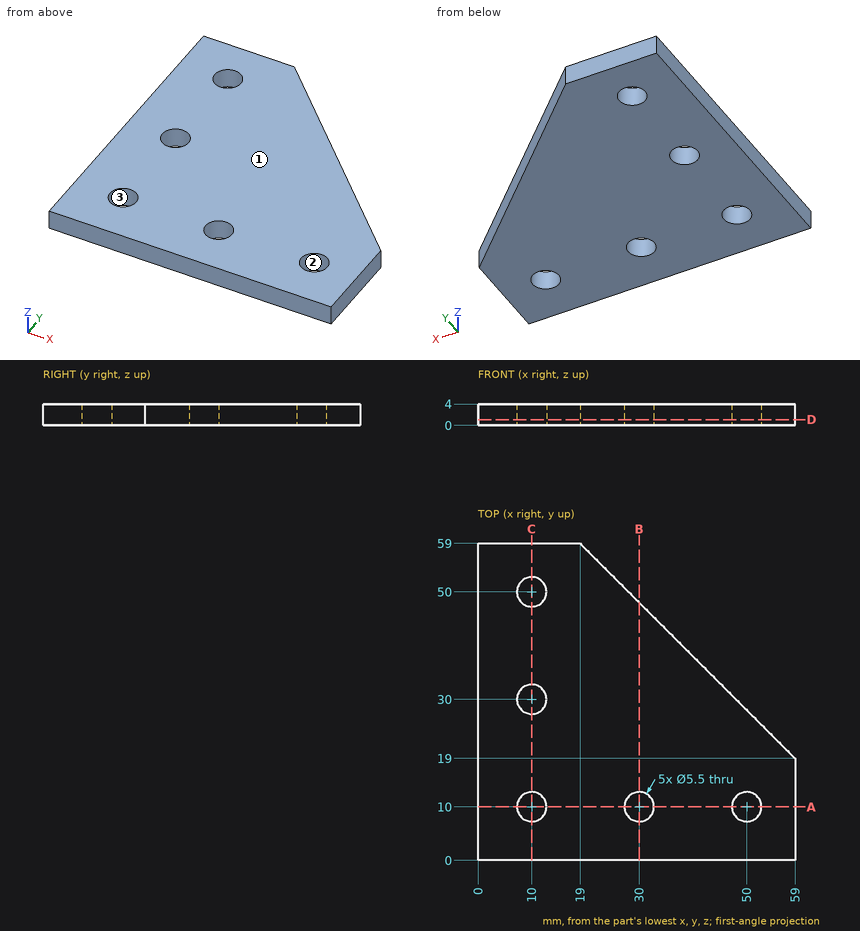
Here's the drawing with two shaded views (mm, measured from the low corner). I have some questions. Give positions to 0.01 mm unless a question says otherwise; leave off trailing zeros. Loops run counter-clockwise (first coordinate to the right, second up) from the corner with the lowest first, then second, coordinate; pieces in that order, holes last. Notation, with made-up numbers: (59, 37.25) - (96, 37.25) arc R24 cw to (96, 72.25) - close; hole circle Ø2 at (55.25, 82). An arc over 180 degrees is marked (long way). One line per item, written item: value.
(1) If we section it at B-B, the plane x = 30: List the corners of the cut face in (y, z) for me, plus the area to 3 significant figures.
Verdict:
outline: (0, 0) - (7.25, 0) - (7.25, 4) - (0, 4) - close; (12.75, 0) - (48, 0) - (48, 4) - (12.75, 4) - close
area: 170 mm^2
(2) If we mould it in two halves opening along X, with no side actions, what happens to the marked faces 1, 2 and 3? For each: released by +X, released by -X, zero draft, split by the parting line, or undercut.
Verdict:
face 1: zero draft
face 2: undercut
face 3: undercut
(3) I'm going to push flat-ended pins straight in: pin 1 (2 mm diameter, centred on x = 46, z = 2.5, fed in from -Y); pin 2 (4.5 mm diameter, centred on x = 30, y = 10, fed in from -Z). Where does each tip first touch, or does it pass through?
Verdict:
pin 1: y = 0
pin 2: through
(4) If we section it at A-A, the plane y = 10: List the corners of the cut face in (x, z) for me, plus the area to 3 significant figures.
Verdict:
outline: (0, 0) - (7.25, 0) - (7.25, 4) - (0, 4) - close; (12.75, 0) - (27.25, 0) - (27.25, 4) - (12.75, 4) - close; (32.75, 0) - (47.25, 0) - (47.25, 4) - (32.75, 4) - close; (52.75, 0) - (59, 0) - (59, 4) - (52.75, 4) - close
area: 170 mm^2
(5) If we section it at D-D, the plane z = 1.1: List the corners of the cut face in (x, y) for me.
Verdict:
outline: (0, 0) - (59, 0) - (59, 19) - (19, 59) - (0, 59) - close; hole circle Ø5.5 at (10, 10); hole circle Ø5.5 at (10, 30); hole circle Ø5.5 at (10, 50); hole circle Ø5.5 at (30, 10); hole circle Ø5.5 at (50, 10)
(6) I need wall thicknesses on line 1 along Y through (x, z) = (10, 1.5); line 2 along Y through (x, z) = (9, 3.4); line 3 along Y through (x, z) = (50, 2.55). Which ranges of each line are inside material? Lowest first, please.
Verdict:
line 1: 0 to 7.25, 12.75 to 27.25, 32.75 to 47.25, 52.75 to 59
line 2: 0 to 7.44, 12.56 to 27.44, 32.56 to 47.44, 52.56 to 59
line 3: 0 to 7.25, 12.75 to 28
